```python
from build123d import *

# Parameters (mm, degrees)
SKETCH1_W           = 53.4573
SKETCH1_H           = 13
SKETCH1_R           = 4.2
BOSS_EXTRUDE1_DEPTH = 50.3
BOSS_EXTRUDE2_START = -15
SKETCH3_R           = 4.2
BOSS_EXTRUDE2_DEPTH = 15
SKETCH8_W           = 15.5
SKETCH8_H           = 13
BOSS_EXTRUDE3_DEPTH = 10.6
CHAMFER1_SIZE       = 10.6
SKETCH5_R           = 3
SKETCH5_R_2         = 4
CUT_EXTRUDE1_DEPTH  = 76.366988286
CUT_EXTRUDE2_DEPTH  = 5.3
BOSS_EXTRUDE4_DEPTH = 10
CUT_EXTRUDE3_DEPTH  = 1
SKETCH13_W          = 21.695080859
SKETCH13_H          = 9.09610943
CUT_EXTRUDE4_DEPTH  = 3
SKETCH16_R          = 1.65
CUT_EXTRUDE5_DEPTH  = 59.425257644
SKETCH17_R          = 7.3
CUT_EXTRUDE6_DEPTH  = 10.5
SKETCH15_W          = 4
SKETCH15_H          = 8
CUT_EXTRUDE7_DEPTH  = 60.472016368
SKETCH18_R          = 8.3
CUT_EXTRUDE8_DEPTH  = 1.2
SKETCH21_R          = 1.65
CUT_EXTRUDE9_DEPTH  = 60.472016368
CUT_EXTRUDE10_DEPTH = 2.6
CUT_EXTRUDE11_START = -1
CUT_EXTRUDE11_DEPTH = 10
BOSS_EXTRUDE5_DEPTH = 13
CUT_EXTRUDE12_START = 10
SKETCH27_R          = 3
CUT_EXTRUDE12_DEPTH = 10
BOSS_EXTRUDE7_DEPTH = 1.5
CUT_EXTRUDE13_REACH = 81.875
CHAMFER2_SIZE       = 0.5


# Read off the part's stored shape, not the designer's step: Cut-Extrude11
with BuildPart() as part:
    # Sketch1 → Boss-Extrude1 (new body)
    with BuildSketch(Plane.XY):
        Rectangle(SKETCH1_W, SKETCH1_H)
        with Locations(Location((-20, 0, 0), (0, 0, 180))):
            Circle(SKETCH1_R, mode=Mode.SUBTRACT)
        with Locations(Location((20, 0, 0), (0, 0, 180))):
            Circle(SKETCH1_R, mode=Mode.SUBTRACT)
    extrude(amount=BOSS_EXTRUDE1_DEPTH)

    # Sketch3 → Boss-Extrude2 (add)
    with BuildSketch(Plane.XY.offset(50.3).offset(BOSS_EXTRUDE2_START)):
        with Locations(Location((-20, 0, 0), (0, 0, 180))):
            Circle(SKETCH3_R)
        with Locations(Location((20, 0, 0), (0, 0, 180))):
            Circle(SKETCH3_R)
    extrude(amount=BOSS_EXTRUDE2_DEPTH)

    # Sketch8 → Boss-Extrude3 (add)
    with BuildSketch(Plane(origin=(0, 6.5, 0), x_dir=(1, 0, 0), z_dir=(0, 1, 0))):
        with Locations((0, -6.5)):
            Rectangle(SKETCH8_W, SKETCH8_H)
    extrude(amount=BOSS_EXTRUDE3_DEPTH)

    # Chamfer1
    chamfer1_edges = [part.edges().sort_by_distance(p)[0] for p in [
        (7.75, 6.5, 6.5),
        (-7.75, 6.5, 6.5),
    ]]
    chamfer(chamfer1_edges, length=CHAMFER1_SIZE - 0.0001)  # a hair under: the kernel refuses the full size

    # Sketch5 → Cut-Extrude1 (cut, through all)
    with BuildSketch(Plane.ZY.offset(26.72865)):
        with Locations(Location((6.5, 12.5, 0), (0, 0, 270))):
            Circle(SKETCH5_R)
        with Locations((36.5, 12.5)):
            Circle(SKETCH5_R_2)
    extrude(amount=-CUT_EXTRUDE1_DEPTH, mode=Mode.SUBTRACT)

    # Sketch10 → Cut-Extrude2 (cut)
    with BuildSketch(Plane.ZY):
        Polygon((2.516283143, 14.8), (2.516283143, 17.1), (10.483716857, 17.1), (10.483716857, 14.8), (10.483716857, 10.2), (6.5, 7.9), (2.516283143, 10.2), align=None)
    cut_extrude2 = extrude(amount=-CUT_EXTRUDE2_DEPTH, mode=Mode.SUBTRACT)

    # Mirror1: Cut-Extrude2 across plane
    add(cut_extrude2.mirror(Plane.ZY), mode=Mode.SUBTRACT)

    # Sketch11 → Boss-Extrude4 (add)
    with BuildSketch(Plane.ZY.offset(26.72865)):
        with BuildLine():
            Line((33.035176772, 15.964823228), (29.509293572, 15.964823228))
            Line((29.509293572, 15.964823228), (22.7, 6.5))
            Line((22.7, 6.5), (50.3, 6.5))
            Line((50.3, 6.5), (43.490706428, 15.964823228))
            Line((43.490706428, 15.964823228), (39.964823228, 15.964823228))
            ThreePointArc((39.964823228, 15.964823228), (36.5, 7.6), (33.035176772, 15.964823228))
        make_face()
    boss_extrude4 = extrude(amount=-BOSS_EXTRUDE4_DEPTH)

    # Sketch12 → Cut-Extrude3 (cut)
    with BuildSketch(Plane.ZY.offset(24.72865)):
        with BuildLine():
            Line((30.15, 12.5), (30.15, 21.960655534))
            Line((30.15, 21.960655534), (42.85, 21.960655534))
            Line((42.85, 21.960655534), (42.85, 12.5))
            ThreePointArc((42.85, 12.5), (36.5, 6.15), (30.15, 12.5))
        make_face()
    cut_extrude3 = extrude(amount=-CUT_EXTRUDE3_DEPTH, mode=Mode.SUBTRACT)

    # Sketch13 → Cut-Extrude4 (cut)
    with BuildSketch(Plane.ZY.offset(26.72865)):
        with Locations((35.453328021, 17.048054715)):
            Rectangle(SKETCH13_W, SKETCH13_H)
    cut_extrude4 = extrude(amount=-CUT_EXTRUDE4_DEPTH, mode=Mode.SUBTRACT)

    # Mirror2: Boss-Extrude4, Cut-Extrude3, Cut-Extrude4 across plane
    add(boss_extrude4.mirror(Plane.ZY))
    add(cut_extrude3.mirror(Plane.ZY), mode=Mode.SUBTRACT)
    add(cut_extrude4.mirror(Plane.ZY), mode=Mode.SUBTRACT)

    # Sketch16 → Cut-Extrude5 (cut, through all)
    with BuildSketch(Plane(origin=(0, 6.5, 0), x_dir=(1, 0, 0), z_dir=(0, 1, 0))):
        with Locations(Location((0, -29.3, 0), (0, 0, 180))):
            Circle(SKETCH16_R)
    extrude(amount=-CUT_EXTRUDE5_DEPTH, mode=Mode.SUBTRACT)

    # Sketch17 → Cut-Extrude6 (cut)
    with BuildSketch(Plane(origin=(0, 6.5, 0), x_dir=(1, 0, 0), z_dir=(0, 1, 0))):
        with Locations(Location((0, -29.3, 0), (0, 0, 180))):
            Circle(SKETCH17_R)
    extrude(amount=-CUT_EXTRUDE6_DEPTH, mode=Mode.SUBTRACT)

    # Sketch15 → Cut-Extrude7 (cut, through all)
    with BuildSketch(Plane(origin=(0, 0, 0), x_dir=(-1, 0, 0), z_dir=(0, 0, -1))):
        with Locations((-5.3, 0)):
            Rectangle(SKETCH15_W, SKETCH15_H)
    cut_extrude7 = extrude(amount=-CUT_EXTRUDE7_DEPTH, mode=Mode.SUBTRACT)

    # Mirror3: Cut-Extrude7 across plane
    add(cut_extrude7.mirror(Plane.ZY), mode=Mode.SUBTRACT)

    # Sketch18 → Cut-Extrude8 (cut)
    with BuildSketch(Plane(origin=(0, 6.5, 0), x_dir=(1, 0, 0), z_dir=(0, 1, 0))):
        with Locations(Location((0, -29.3, 0), (0, 0, 180))):
            Circle(SKETCH18_R)
    extrude(amount=-CUT_EXTRUDE8_DEPTH, mode=Mode.SUBTRACT)

    # Sketch20 → Revolve1 (revolve)
    with BuildSketch(Plane.ZY, mode=Mode.PRIVATE) as revolve1_sk:
        Polygon((30.95, -4), (30.95, -2), (31.95, -2), (33.95, -4), align=None)
    revolve(revolve1_sk.sketch.rotate(Axis((0, -4, 29.3), (0, 1, 0)), 270), axis=Axis((0, -4, 29.3), (0, 1, 0)))

    # Sketch21 → Cut-Extrude9 (cut, through all)
    with BuildSketch(Plane.XY.offset(50.3)):
        with Locations((20, 0)):
            Circle(SKETCH21_R)
        with Locations((-20, 0)):
            Circle(SKETCH21_R)
    extrude(amount=-CUT_EXTRUDE9_DEPTH, mode=Mode.SUBTRACT)

    # Sketch22 → Cut-Extrude10 (cut)
    with BuildSketch(Plane.XY.offset(46.3)):
        Polygon((-22.901185103, 1.227039119), (-22.901185103, 2.802039119), (-17.098814897, 2.802039119), (-17.098814897, 1.413894196), (-17.098814897, -1.675), (-17.098814897, -7.277237341), (-22.901185103, -7.277237341), (-22.901185103, -1.675), align=None)
    cut_extrude10 = extrude(amount=-CUT_EXTRUDE10_DEPTH, mode=Mode.SUBTRACT)

    # Mirror4: Cut-Extrude10 across plane
    add(cut_extrude10.mirror(Plane.ZY), mode=Mode.SUBTRACT)

    # Cut-Extrude11 outline → Cut-Extrude11 (cut)
    with BuildSketch(Plane(origin=(0, -4, 0), x_dir=(1, 0, 0), z_dir=(0, 1, 0)).offset(CUT_EXTRUDE11_START)):
        with BuildLine():
            ThreePointArc((3.3, -20.391577019), (5.485502581, -21.543759839), (7.3, -23.220526339))
            Line((7.3, -23.220526339), (7.3, -2))
            Line((7.3, -2), (3.3, -2))
            Line((3.3, -2), (3.3, -20.391577019))
        make_face()
        with BuildLine():
            Line((-7.3, -2), (-7.3, -23.220526339))
            ThreePointArc((-7.3, -23.220526339), (-5.485502581, -21.543759839), (-3.3, -20.391577019))
            Line((-3.3, -20.391577019), (-3.3, -2))
            Line((-3.3, -2), (-7.3, -2))
        make_face()
    extrude(amount=CUT_EXTRUDE11_DEPTH, mode=Mode.SUBTRACT)

    # Sketch26 → Boss-Extrude5 (add)
    with BuildSketch(Plane(origin=(0, 0, 0), x_dir=(-1, 0, 0), z_dir=(0, 0, -1))):
        Polygon((24.4510146, 6.5), (26.72865, 6.5), (36.02865, 23.567646595), (36.02865, 31.5), (34.02865, 31.5), (34.02865, 24.077171637), align=None)
    extrude(amount=-BOSS_EXTRUDE5_DEPTH)

    # Sketch27 → Cut-Extrude12 (cut)
    with BuildSketch(Plane.ZY.offset(26.72865).offset(CUT_EXTRUDE12_START)):
        with Locations(Location((6.5, 12.5, 0), (0, 0, 270))):
            Circle(SKETCH27_R)
    extrude(amount=-CUT_EXTRUDE12_DEPTH, mode=Mode.SUBTRACT)

    # Sketch29 → Boss-Extrude7 (add)
    with BuildSketch(Plane(origin=(0, 0, 0), x_dir=(-1, 0, 0), z_dir=(0, 0, -1))):
        Polygon((26.72865, -6.5), (36.02865, 23.567646595), (26.72865, 6.5), align=None)
    boss_extrude7 = extrude(amount=-BOSS_EXTRUDE7_DEPTH)

    # Mirror5: Boss-Extrude7 across plane
    add(boss_extrude7.mirror(Plane(origin=(0, 0, 6.5), x_dir=(1, 0, 0), z_dir=(0, 0, -1))))

    # Sketch30 → Cut-Extrude13 (cut, up to next)
    with BuildSketch(Plane.ZY.offset(26.72865), mode=Mode.PRIVATE) as cut_extrude13_sk1:
        with BuildLine():
            Line((8.8848588, 10.679986675), (4.1151412, 10.679986675))
            ThreePointArc((4.1151412, 10.679986675), (6.5, 9.5), (8.8848588, 10.679986675))
        make_face()
    cut_extrude13_tool1 = extrude(cut_extrude13_sk1.sketch, amount=-CUT_EXTRUDE13_REACH, mode=Mode.PRIVATE) & part.part
    add(cut_extrude13_tool1.solids().sort_by_distance((-26.72865, 10.199004, 6.5))[0], mode=Mode.SUBTRACT)

    # Chamfer2
    chamfer2_edges = [part.edges().sort_by_distance(p)[0] for p in [
        (1.65, -6.5, 29.3),
        (-17.098814897, -6.5, 45),
        (-22.901185103, -6.5, 45),
        (-20, -6.5, 43.7),
        (-20, -6.5, 46.3),
        (22.901185103, -6.5, 45),
        (17.098814897, -6.5, 45),
        (20, -6.5, 43.7),
        (20, -6.5, 46.3),
    ]]
    chamfer(chamfer2_edges, length=CHAMFER2_SIZE)


solid = part.part
```
Build history of the part. All positions in model axes, mm. A direction names the side the tool comes from. Give positions to 0.01 mm unless a question says otherwise; leave off trailing zeros. Order: outer loops, then holes, each group sorted by start corner. A loop starts at its lowest first (then second) coordinate and runs counter-clockwise, first axis right, second up. Notation, with made-up numbers: M 10,6.5 L 25,6.5 A19 cw 25,37.5 Z; hole C -32.75,30 d1. An arc over 180 degrees is marked long. Write item = value, one per line. Start each with the question number.
(1) Slice it at A-A on x = -20. Write the cut outline in (y, z), plus the area to 3 significant figures.
(2) Slice it at B-B on y = 0. State how many separate pieces and enclosed holes the cut face has, plus the area to 3 significant figures.
(3) Slice it at D-D on y = 18.5. Write the cut outline in (x, z), plus the area to 3 significant figures.
(4) Slice it at C-C on x = -11. Write the cut outline in (y, z).
(5) Which spindle directions (+Z, -Z, +X, -X, +Y, -Y) get a long thin tool onto all of the face, cutting with end or side? Do faces 3 (the flat face through (-32.347, 16.811, 6.43)), 4 (the flat face through (-24.729, 7, 37)), 5 (the flat face through (-20, -3, 43.7)). Say none if no direction does.
(6) Pin check, flat tips, straight feed: pin 1 Ø5 at (x, z) = (12, 11) entering from +Y; pin 2 Ø5.5 at (x, y) = (20, 0) entering from -Z; pin 3 Ø1.7 at (x, y) = (20.5, -1.5) entering from +Z; pin 4 Ø2 at (y, z) = (19.5, 7) entering from +X. Stop position of each tip, or through.
(7) Probe L1, parallel to X at y = 3.5, z = 45; L2, parallel to Z at x = 0, y = 1; L3, parallel to X at y = -0.5, z = 29.3. List the from-to ranges inside material, lowest first. Write a range as [from, to].
(8) Two-plate mould, pull along Z, no slides. Class faces 1 (the cylindrical face through (-20.278, 7.603, 36.662)), 2 (the flat face through (25, 12.5, 44)): released by +Z, released by -Z, zero draft, split by the parting line, or undercut.
Responses:
q1.outline = M -6.5,0 L -4.2,0 L -4.2,35.3 L -1.65,35.3 L -1.65,43.7 L -6,43.7 L -6.5,43.2 Z; M -6.5,46.8 L -6,46.3 L -1.65,46.3 L -1.65,50.3 L -6.5,50.3 Z; M 1.65,35.3 L 4.2,35.3 L 4.2,0 L 6.5,0 L 6.5,22.7 L 15.96,29.51 L 15.96,33.04 A4.9 cw long 15.96,39.96 L 15.96,43.49 L 6.5,50.3 L 1.65,50.3 L 1.65,46.3 L 2.8,46.3 L 2.8,43.7 L 1.65,43.7 Z
q1.area = 420 mm2
q2.separate_pieces = 6
q2.enclosed_holes = 0
q2.area = 1,490 mm2
q3.outline = M -34.46,0 L -30.99,0 L -30.99,13 L -34.46,13 L -34.46,11.5 L -33.27,11.5 L -33.27,1.5 L -34.46,1.5 Z
q3.area = 33.2 mm2
q4.outline = M -6.5,0 L 13.85,0 L 13.85,3.82 A3 cw long 13.85,9.18 L 13.85,13 L 6.5,13 L 6.5,50.3 L -6.5,50.3 Z
q5.face_3 = -X, -Y
q5.face_4 = +Y
q5.face_5 = -Y
q6.pin_1 = 15.35
q6.pin_2 = 35.3
q6.pin_3 = 50.3
q6.pin_4 = -30.99
q7.L1 = [-26.73, -7.3], [-3.3, 3.3], [7.3, 26.73]
q7.L2 = [0, 22], [36.6, 50.3]
q7.L3 = [-26.73, -24.17], [-15.83, -7.3], [7.3, 15.83], [24.17, 26.73]
q8.face_1 = undercut
q8.face_2 = zero draft
